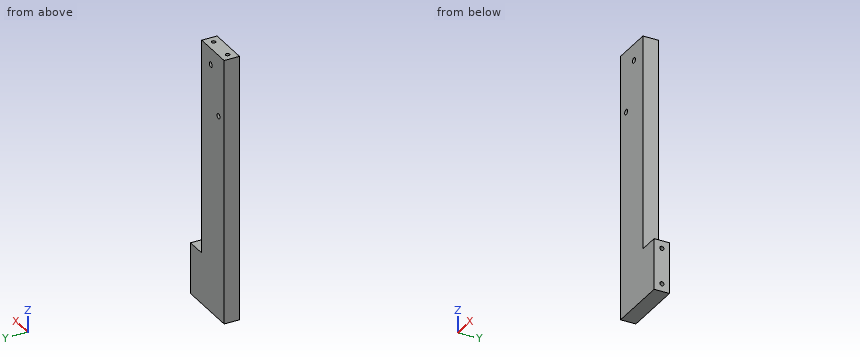
from build123d import *

# Parameters (mm, degrees)
F0_W      = 76.2
F0_H      = 330.2
F1_DEPTH  = 19.05
F2_W      = 25.4
F2_H      = 266.7
F3_DEPTH  = 19.051
F4_R      = 3.2639
F5_DEPTH  = 19.051
F6_R      = 3.2639
F7_DEPTH  = 19.051
F9_D      = 5.1054
F9_DEPTH  = 16.51
F9_TIP    = 1.5338169022
F11_D     = 5.1054
F11_DEPTH = 16.51
F11_TIP   = 1.5338169022


with BuildPart() as f1:
    # F0 (on Front) → F1 (new body)
    with BuildSketch(Plane.XZ):
        with Locations((38.1, 165.1)):
            Rectangle(F0_W, F0_H)
    extrude(amount=F1_DEPTH)

    # F2 (on face) → F3 (cut, through all)
    with BuildSketch(Plane.XZ):
        with Locations((63.5, 196.85)):
            Rectangle(F2_W, F2_H)
    extrude(amount=F3_DEPTH, mode=Mode.SUBTRACT)

    # F4 (on face) → F5 (cut, through all)
    with BuildSketch(Plane.XZ.offset(19.05)):
        with Locations((12.7, 254)):
            Circle(F4_R)
    extrude(amount=-F5_DEPTH, mode=Mode.SUBTRACT)

    # F6 (on face) → F7 (cut, through all)
    with BuildSketch(Plane.XZ.offset(19.05)):
        with Locations((30.4351865955, 309.8351865955)):
            Circle(F6_R)
    extrude(amount=-F7_DEPTH, mode=Mode.SUBTRACT)

    # F9
    with Locations(Plane.XY.offset(330.2)):
        with Locations((9.525, -9.525), (41.275, -9.525)):
            Hole(F9_D / 2, depth=F9_DEPTH)
            with Locations((0, 0, -(F9_DEPTH + F9_TIP / 2))):  # 118° drill point
                Cone(0, F9_D / 2, F9_TIP, mode=Mode.SUBTRACT)

    # F11
    with Locations(Plane.YZ.offset(76.2)):
        with Locations((-9.525, 53.975), (-9.525, 9.525)):
            Hole(F11_D / 2, depth=F11_DEPTH)
            with Locations((0, 0, -(F11_DEPTH + F11_TIP / 2))):  # 118° drill point
                Cone(0, F11_D / 2, F11_TIP, mode=Mode.SUBTRACT)


solid = f1.part
Can you work these out from the model? Positions are in its coordinate system, mm. Coordinates: 2 decimals unless noted, no trailing zeros. Write each loop counter-clockwise with the first axis right and the second up, starting at its lowest first coordinate (ties: lowest second). Pieces come first, ordered by that corner, then holes. Notation, with made-up numbers: (48.5, 44.25) -> (103.5, 44.25) arc R20 ccw to (103.5, 78.25) -> close; hole circle Ø4 at (20, 37). An arc over 180 degrees is marked (long way). Answer as CSV lines item,"result".
1) If we section it at A-A on z = 254: Please give me the cut outline in (x, y), then the cut area to 3 significant figures.
Check result:
outline,"(0, -19.05) -> (9.44, -19.05) -> (9.44, 0) -> (0, 0) -> close; (15.96, -19.05) -> (50.8, -19.05) -> (50.8, 0) -> (15.96, 0) -> close"
area,"843 mm²"
2) If we section it at C-C on x = 64: Please give me the cut outline in (y, z) (3 decimals), then the cut area to 3 significant figures.
Check result:
outline,"(-19.05, 0) -> (0, 0) -> (0, 63.5) -> (-19.05, 63.5) -> close; hole circle Ø5.105 at (-9.525, 9.525); hole circle Ø5.105 at (-9.525, 53.975)"
area,"1,170 mm²"
3) If I drill on line 1 (Z direction, x = 12.7, y = -8.5); line 2 (X direction, y = -11, z = 316); line 3 (X direction, y = -12, z = 254), over which ranges is the centre line in solid material (lowest first)? Write a range as from..to.
Check result:
line 1,"0..250.74, 257.26..330.2"
line 2,"0..7.44, 11.61..39.19, 43.36..50.8"
line 3,"0..9.44, 15.96..50.8"
4) If we section it at B-B on y = -4.25: Please give me the cut outline in (x, z).
Check result:
outline,"(0, 0) -> (76.2, 0) -> (76.2, 63.5) -> (50.8, 63.5) -> (50.8, 330.2) -> (0, 330.2) -> close; hole circle Ø6.53 at (12.7, 254); hole circle Ø6.53 at (30.44, 309.84)"
5) Will these pins go through, and if not, where does the flat tip stop? P1, Ø1.5, axis at y = -8, z = 219.5, coming from the +X side; P2, Ø5.5, axis at x = 58, y = -9, coming from the +Z side.
Check result:
P1,"x = 50.8"
P2,"z = 63.5"
